from build123d import *

# Parameters (mm, degrees)
SKETCH1_W           = 15
SKETCH1_H           = 15
BOSS_EXTRUDE1_DEPTH = 5
BOSS_EXTRUDE2_DEPTH = 5
BOSS_EXTRUDE2_TAPER = 1
SKETCH3_R           = 4
BOSS_EXTRUDE3_DEPTH = 10


with BuildPart() as part:
    # Sketch1 → Boss-Extrude1 (new body)
    with BuildSketch(Plane(origin=(0, 0, 0), x_dir=(1, 0, 0), z_dir=(0, 1, 0))):
        Rectangle(SKETCH1_W, SKETCH1_H)
    extrude(amount=BOSS_EXTRUDE1_DEPTH)

    # Sketch2 → Boss-Extrude2 (add)
    with BuildSketch(Plane(origin=(0, 5, 0), x_dir=(1, 0, 0), z_dir=(0, 1, 0))):
        with BuildLine():
            Line((-4.999500013, -0.049742391), (-0.049747468, -4.999494936))
            Line((-0.049747468, -4.999494936), (4.949747468, 0))
            ThreePointArc((4.949747468, 0), (4.924747439, 4.974497472), (-0.049247481, 4.89949991))
            ThreePointArc((-0.049247481, 4.89949991), (-4.999247442, 4.900257622), (-4.999500013, -0.049742391))
        make_face()
    extrude(amount=BOSS_EXTRUDE2_DEPTH, taper=BOSS_EXTRUDE2_TAPER)

    # Sketch3 → Boss-Extrude3 (add)
    with BuildSketch(Plane.XZ):
        with Locations(Location((0, 0, 0), (0, 0, 270))):
            Circle(SKETCH3_R)
    extrude(amount=BOSS_EXTRUDE3_DEPTH)


solid = part.part
Here's how the part is built. I have some questions about the finished solid (model axes, mm). A direction names the side the tool comes from. Give positions to 0.01 mm unless a question says otherwise; leave off trailing zeros. Write each loop counter-clockwise with the first axis right and the second up, starting at its lowest first coordinate (ties: lowest second). Pieces come first, ordered by that corner, then holes. Notation, with made-up numbers: (80.25, -18) -> (98.25, -18) arc R33 ccw to (98.25, 20) -> close; hole circle Ø6 at (73, 27). An arc over 180 degrees is marked (long way). Use one line per item in the form item = value. Start each with the question number.
1. If I drill on L1, parallel to Y at x = 4.25, z = -5; L2, parallel to Y at x = -6.5, z = 5.75; L3, parallel to X at y = 5.5, z = -5.5, over which ranges is the centre line in solid material (lowest first)?
2. Thinking about a two-plate mould opening in Y: for faces 1 (the face through (0, 10, -1)), 2 (the face through (7.5, 2, 0)), 3 (the face through (-3, 0, -3)), which applies, +Y half, -Y half, draft (parallel to the pull), parting line (faces both ways), or undercut?
3. Imagine slicing it at A-A on z = -6.25. List the corners of the cut face in (x, y) for me, plus the area to 3 significant figures.
4. On a 3-axis mill with a long thin cutter (end or side, diameter ignored), from which of +Z, -Z, +X, -X, +Y, -Y can I reach the whole of each face in a straight line? I mean faces 4 (the face through (0, -10, 0)), 5 (the face through (-3, 5, 3)), 6 (the face through (-3.905, -4.93, 0.867)). Say none if no direction works.
5. Will this pin go through, and if not, where does the flat tip stop? pin 1 Ø8 at (x, y) = (-6, -5) entering from +Z.
Entries:
q1.L1 = 0 to 10
q1.L2 = 0 to 5
q1.L3 = -4.18 to -0.87, 0.73 to 4.22
q2.face_1 = +Y half
q2.face_2 = draft
q2.face_3 = -Y half
q3.outline = (-7.5, 0) -> (7.5, 0) -> (7.5, 5) -> (-7.5, 5) -> close
q3.area = 75.0 mm²
q4.face_4 = +Z, -Z, +X, -X, -Y
q4.face_5 = +Y
q4.face_6 = -Y
q5.pin_1 = 3.46
